Source: CAD feature listing. Evaluate the final solid. Frame: model axes, mm. Face numbers are marked on the shaded views. A direction names the side the tool comes from. Round coordinates to 2 decimals unless told otherwise and drop trailing zeros. Loops run counter-clockwise (first coordinate to the right, second up) from the corner with the lowest first, then second, coordinate; pieces in that order, holes last.
Item 1: First-contact query: P1, Ø5, axis at y = 7.5, z = 12, coming from the +X side (3 decimals); P2, Ø8, axis at x = 20, y = 22, coming from the -Z side; P3, Ø3, axis at x = 9, z = -10.5, coming from the +Y side; P4, Ø7, axis at x = 18.65, y = 50.82, coming from the +Z side. Flat tips, straight axial feed; report the tip coordinate or a pass-through.
Item 2: Section query A-A on x = 18.65. Return loops of the section in (y, z) (3 decimals), then the cut area to 3 significant figures.
Item 3: Ray query, L1, parallel to X at y = 50.82, z = -6.2; L2, parallel to Z at x = 11, y = 7.5 (3 decimals); L3, parallel to Y at x = 45, z = 6. Return the intervals inside material, ascending.
Item 4: Section query B-B on y = 14. Return loops of the section in (x, z) (3 decimals), then the cut area to 3 significant figures.
Item 5: Section query D-D on y = 50.82. Return loops of the section in (x, z) (3 decimals).
Item 6: Access query for the marked faces 1, 2 and 3. Directions: +Z, -Z, +X, -X, +Y, -Y. A direction counts if a zero-diameter tool reaches every point of the face in a straight line with its end or side. Return the directions, or none.
Item 7: Section query C-C on x = 8. Return loops of the section in (y, z) (3 decimals), then the cut area to 3 significant figures.
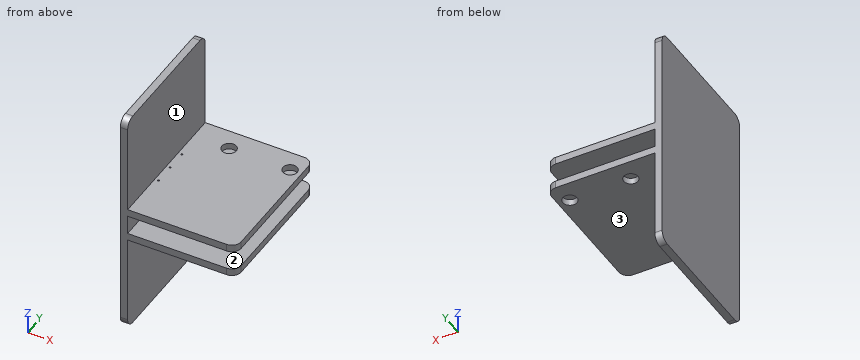
```python
from build123d import *

# Parameters (mm, degrees)
BOSS_EXTRUDE1_DEPTH = 60
SKETCH3_R           = 3.1
CUT_EXTRUDE1_DEPTH  = 2.7
CUT_EXTRUDE2_START  = -2.7
SKETCH4_R           = 3.1
CUT_EXTRUDE2_DEPTH  = 2.7
FILLET1_R           = 4
CUT_EXTRUDE3_REACH  = 81.474
SKETCH5_R           = 0.375
SKETCH6_W           = 3.175
SKETCH6_H           = 60
BOSS_EXTRUDE2_DEPTH = 42.65
SKETCH7_W           = 3.175
SKETCH7_H           = 60
BOSS_EXTRUDE3_DEPTH = 42.65
FILLET2_R           = 4


with BuildPart() as part:
    # Sketch1 → Boss-Extrude1 (new body)
    with BuildSketch(Plane(origin=(0, 0, 0), x_dir=(1, 0, 0), z_dir=(0, 1, 0))):
        Polygon((0, 7.35), (0, -7.35), (50, -7.35), (50, -4.175), (3.175, -4.175), (3.175, 4.175), (50, 4.175), (50, 7.35), align=None)
    extrude(amount=BOSS_EXTRUDE1_DEPTH)

    # Sketch3 → Cut-Extrude1 (cut)
    with BuildSketch(Plane.XY.offset(7.35)):
        with Locations((45, 50.82)):
            Circle(SKETCH3_R)
        with Locations((18.65, 50.82)):
            Circle(SKETCH3_R)
    extrude(amount=-CUT_EXTRUDE1_DEPTH, mode=Mode.SUBTRACT)

    # Sketch4 → Cut-Extrude2 (cut)
    with BuildSketch(Plane(origin=(0, 0, -7.35), x_dir=(-1, 0, 0), z_dir=(0, 0, -1)).offset(CUT_EXTRUDE2_START)):
        with Locations(Location((-45, 50.82, 0), (0, 0, 180))):
            Circle(SKETCH4_R)
        with Locations(Location((-18.65, 50.82, 0), (0, 0, 180))):
            Circle(SKETCH4_R)
    extrude(amount=CUT_EXTRUDE2_DEPTH, mode=Mode.SUBTRACT)

    # Fillet1
    fillet1_edges = [part.edges().sort_by_distance(p)[0] for p in [
        (50, 0, 5.7625),
        (50, 60, -5.7625),
        (50, 60, 5.7625),
        (50, 0, -5.7625),
    ]]
    fillet(fillet1_edges, radius=FILLET1_R)

    # Cut-Extrude3: up to this face of the body (flat: up to its plane)
    cut_extrude3_end = Plane(part.part.faces().sort_by_distance((24.80303516, 29.571344164, -7.35))[0])
    # Sketch5 → Cut-Extrude3 (cut, up to the picked face)
    with BuildSketch(Plane.XY.offset(7.35), mode=Mode.PRIVATE) as cut_extrude3_sk1:
        with Locations((4.779169586, 21)):
            Circle(SKETCH5_R)
    cut_extrude3_tool1 = split(extrude(cut_extrude3_sk1.sketch, amount=-CUT_EXTRUDE3_REACH, mode=Mode.PRIVATE), bisect_by=cut_extrude3_end, keep=Keep.BOTH, mode=Mode.PRIVATE)
    # Sketch5 → Cut-Extrude3 (cut, up to the picked face)
    with BuildSketch(Plane.XY.offset(7.35), mode=Mode.PRIVATE) as cut_extrude3_sk2:
        with Locations((4.779169586, 39)):
            Circle(SKETCH5_R)
    cut_extrude3_tool2 = split(extrude(cut_extrude3_sk2.sketch, amount=-CUT_EXTRUDE3_REACH, mode=Mode.PRIVATE), bisect_by=cut_extrude3_end, keep=Keep.BOTH, mode=Mode.PRIVATE)
    # Sketch5 → Cut-Extrude3 (cut, up to the picked face)
    with BuildSketch(Plane.XY.offset(7.35), mode=Mode.PRIVATE) as cut_extrude3_sk3:
        with Locations((4.779169586, 30)):
            Circle(SKETCH5_R)
    cut_extrude3_tool3 = split(extrude(cut_extrude3_sk3.sketch, amount=-CUT_EXTRUDE3_REACH, mode=Mode.PRIVATE), bisect_by=cut_extrude3_end, keep=Keep.BOTH, mode=Mode.PRIVATE)
    add(cut_extrude3_tool1.solids().sort_by(Axis((4.77917, 21, 7.35), (0, 0, -1)))[0], mode=Mode.SUBTRACT)
    add(cut_extrude3_tool2.solids().sort_by(Axis((4.77917, 39, 7.35), (0, 0, -1)))[0], mode=Mode.SUBTRACT)
    add(cut_extrude3_tool3.solids().sort_by(Axis((4.77917, 30, 7.35), (0, 0, -1)))[0], mode=Mode.SUBTRACT)

    # Sketch6 → Boss-Extrude2 (add)
    with BuildSketch(Plane.XY.offset(7.35)):
        with Locations((1.5875, 30)):
            Rectangle(SKETCH6_W, SKETCH6_H)
    extrude(amount=BOSS_EXTRUDE2_DEPTH)

    # Sketch7 → Boss-Extrude3 (add)
    with BuildSketch(Plane(origin=(0, 0, -7.35), x_dir=(-1, 0, 0), z_dir=(0, 0, -1))):
        with Locations((-1.5875, 30)):
            Rectangle(SKETCH7_W, SKETCH7_H)
    extrude(amount=BOSS_EXTRUDE3_DEPTH)

    # Fillet2
    fillet2_edges = [part.edges().sort_by_distance(p)[0] for p in [
        (1.5875, 60, -50),
        (1.5875, 0, -50),
        (1.5875, 0, 50),
        (1.5875, 60, 50),
    ]]
    fillet(fillet2_edges, radius=FILLET2_R)


solid = part.part
```
Data:
1. P1: stops at x = 3.175
1. P2: stops at z = -7.35
1. P3: passes through
1. P4: stops at z = 7.35
2. outline: (0, -7.35) - (47.72, -7.35) - (47.72, -4.65) - (53.92, -4.65) - (53.92, -7.35) - (60, -7.35) - (60, -4.175) - (0, -4.175) - close; (0, 4.175) - (60, 4.175) - (60, 7.35) - (53.92, 7.35) - (53.92, 4.65) - (47.72, 4.65) - (47.72, 7.35) - (0, 7.35) - close
2. area: 348 mm2
3. L1: x = 0 to 15.55, 21.75 to 41.9, 48.1 to 50
3. L2: z = -7.35 to -4.175, 4.175 to 7.35
3. L3: y = 0 to 47.72, 53.92 to 60
4. outline: (0, -50) - (3.175, -50) - (3.175, -7.35) - (50, -7.35) - (50, -4.175) - (3.175, -4.175) - (3.175, 4.175) - (50, 4.175) - (50, 7.35) - (3.175, 7.35) - (3.175, 50) - (0, 50) - close
4. area: 615 mm2
5. outline: (0, -50) - (3.175, -50) - (3.175, -7.35) - (15.55, -7.35) - (15.55, -4.65) - (21.75, -4.65) - (21.75, -7.35) - (41.9, -7.35) - (41.9, -4.65) - (48.1, -4.65) - (48.1, -7.35) - (50, -7.35) - (50, -4.175) - (3.175, -4.175) - (3.175, 4.175) - (50, 4.175) - (50, 7.35) - (48.1, 7.35) - (48.1, 4.65) - (41.9, 4.65) - (41.9, 7.35) - (21.75, 7.35) - (21.75, 4.65) - (15.55, 4.65) - (15.55, 7.35) - (3.175, 7.35) - (3.175, 50) - (0, 50) - close
6. face 1: +Z, +X, +Y, -Y
6. face 2: +X, +Y, -Y
6. face 3: -Z, +X, +Y, -Y
7. outline: (0, -7.35) - (60, -7.35) - (60, -4.175) - (0, -4.175) - close; (0, 4.175) - (60, 4.175) - (60, 7.35) - (0, 7.35) - close
7. area: 381 mm2
